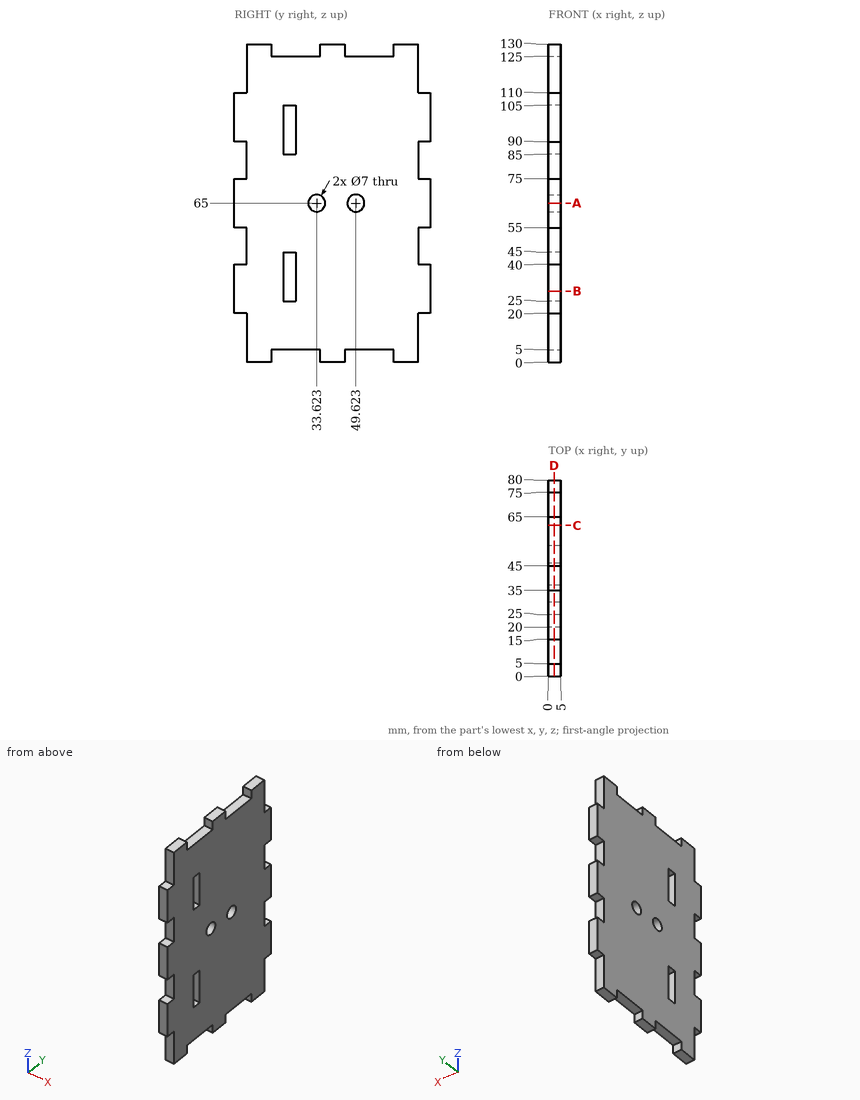
For this review, use the dimensioned drawing (mm, ordinates from the lowest corner) and the shaded views. Coordinates: 2 decimals unless noted, no trailing zeros. Write each loop counter-clockwise with the first axis right and the second up, starting at its lowest first coordinate (ties: lowest second). Pieces come first, ordered by that corner, then holes. Notation, with made-up numbers: (-1.75, -36.5) - (47.25, -36.5) arc R31 ccw to (47.25, -12.5) - close; hole circle Ø7 at (50.5, -27). An arc over 180 degrees is marked (long way). One line per item, written item: value.
1) Add section A-A (z = 65). State the section outline as (x, y) points, plus the area to 3 significant figures.
Answer sheet:
outline: (0, 0) - (5, 0) - (5, 30.12) - (0, 30.12) - close; (0, 37.12) - (5, 37.12) - (5, 46.12) - (0, 46.12) - close; (0, 53.12) - (5, 53.12) - (5, 80) - (0, 80) - close
area: 330 mm2
2) Add section C-C (y = 61.5). State the section outline as (x, z) points.
Answer sheet:
outline: (0, 5) - (5, 5) - (5, 125) - (0, 125) - close
3) Add section B-B (z = 29). State the section outline as (x, y) points.
Answer sheet:
outline: (0, 0) - (5, 0) - (5, 20) - (0, 20) - close; (0, 25) - (5, 25) - (5, 80) - (0, 80) - close
4) Add section D-D (x = 2.4). Give the number of separate pieces and of enclosed holes in the cut face, plus the area to 3 significant figures.
Answer sheet:
separate pieces: 1
enclosed holes: 4
area: 9,020 mm2
5) To check wall thickness, follow probe 1 along Y at (x, z) = (2.05, 65); probe 2 along Z at (x, y) = (0.6, 76); probe 3 along Y at (x, z) = (1.7, 43). State the ranges of each line that lie inside material, in increasing order.
Answer sheet:
probe 1: y = 0 to 30.12, 37.12 to 46.12, 53.12 to 80
probe 2: z = 20 to 40, 55 to 75, 90 to 110
probe 3: y = 5 to 20, 25 to 75
6) Insertion check: pin 1 (1.5 mm diameter, centred on x = 3, y = 3, fed in from -Z); pin 2 (1.5 mm diameter, centred on x = 3, y = 2, fed in from +Z); pin 3 (1.5 mm diameter, centred on x = 2, z = 1.5, fed in from -Y); pin 4 (5.5 mm diameter, centred on y = 49.62, z = 65, fed in from -X) (3 decimals). Each pin has a flat end and moves straight along its axis. Give the tip position at first contact, or say it passes through.
Answer sheet:
pin 1: stops at z = 20
pin 2: stops at z = 110
pin 3: stops at y = 5
pin 4: passes through
